Part model, mm, in its own coordinate system. Coordinates: 2 decimals unless noted, no trailing zeros. Loops run counter-clockwise (first coordinate to the right, second up) from the corner with the lowest first, then second, coordinate; pieces in that order, holes last. Notation, with made-up numbers: M 26,53 L 51,53 A16 cw 51,61 Z; hole C 47,16.25 d6. An arc over 180 degrees is marked long. Use a Markdown table: item, result. Add a question column.
1) Wall check: probe 1 along Z at (x, y) = (10.5, 164.5); probe 2 along X at (y, z) = (593, -11); probe 3 along Z at (x, y) = (-16, 838.5). Give the ranges that are in metal, low to high. Write a range as from..to.
2) Band-saw the part on A-A (z = -11). List the corners of the cut face in (x, y).
3) Pin check, flat tips, straight feed: pin 1 Ø2 at (y, z) = (377, -39.5) entering from +X; pin 2 Ø1.6 at (y, z) = (672.5, -39) entering from -X. Stop position of each tip, or through.
4) Band-saw the part on B-B (y = 124.5). List the corners of the cut face in (x, z), plus the area to 3 significant figures.
from build123d import *

# Parameters (mm, degrees)
EXTRUDE_1_DEPTH = 1025


with BuildPart() as part:
    # Эскиз1 → Вытянуть-Тонкостенный1 (new body)
    with BuildSketch(Plane(origin=(0, 0, 0), x_dir=(1, 0, 0), z_dir=(0, 1, 0))):
        with BuildLine():
            Line((-5, 40), (-15, 40))
            ThreePointArc((-15, 40), (-18.535533906, 38.535533906), (-20, 35))
            Line((-20, 35), (-20, 5))
            ThreePointArc((-20, 5), (-18.535533906, 1.464466094), (-15, 0))
            Line((-15, 0), (15, 0))
            ThreePointArc((15, 0), (18.535533906, 1.464466094), (20, 5))
            Line((20, 5), (20, 35))
            ThreePointArc((20, 35), (18.535533906, 38.535533906), (15, 40))
            Line((15, 40), (5, 40))
            Line((5, 40), (5, 38))
            Line((5, 38), (15, 38))
            ThreePointArc((15, 38), (17.121320344, 37.121320344), (18, 35))
            Line((18, 35), (18, 5))
            ThreePointArc((18, 5), (17.121320344, 2.878679656), (15, 2))
            Line((15, 2), (-15, 2))
            ThreePointArc((-15, 2), (-17.121320344, 2.878679656), (-18, 5))
            Line((-18, 5), (-18, 35))
            ThreePointArc((-18, 35), (-17.121320344, 37.121320344), (-15, 38))
            Line((-15, 38), (-5, 38))
            Line((-5, 38), (-5, 40))
        make_face()
    extrude(amount=EXTRUDE_1_DEPTH)


solid = part.part
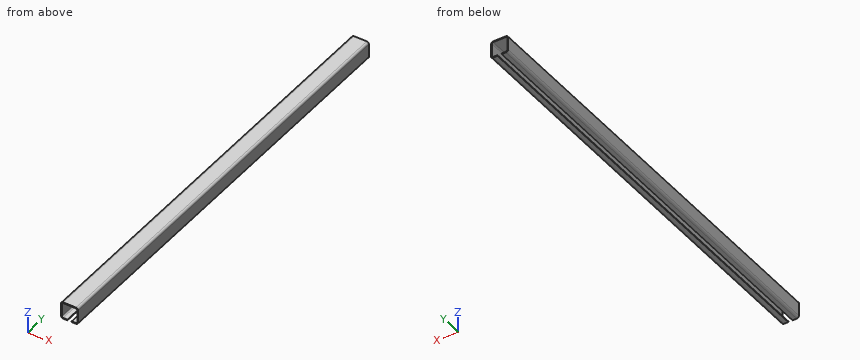
Entries:
| question | item | result |
|---|---|---|
| 1 | probe 1 | -40..-38, -2..0 |
| 1 | probe 2 | -20..-18, 18..20 |
| 1 | probe 3 | -39.9..-37.83, -2.17..-0.1 |
| 2 | outline | M -20,0 L -18,0 L -18,1025 L -20,1025 Z; M 18,0 L 20,0 L 20,1025 L 18,1025 Z |
| 3 | pin 1 | x = 18.57 |
| 3 | pin 2 | x = -18.84 |
| 4 | outline | M -20,-35 A5 ccw -15,-40 L -5,-40 L -5,-38 L -15,-38 A3 cw -18,-35 L -18,-5 A3 cw -15,-2 L 15,-2 A3 cw 18,-5 L 18,-35 A3 cw 15,-38 L 5,-38 L 5,-40 L 15,-40 A5 ccw 20,-35 L 20,-5 A5 ccw 15,0 L -15,0 A5 ccw -20,-5 Z |
| 4 | area | 270 mm2 |
